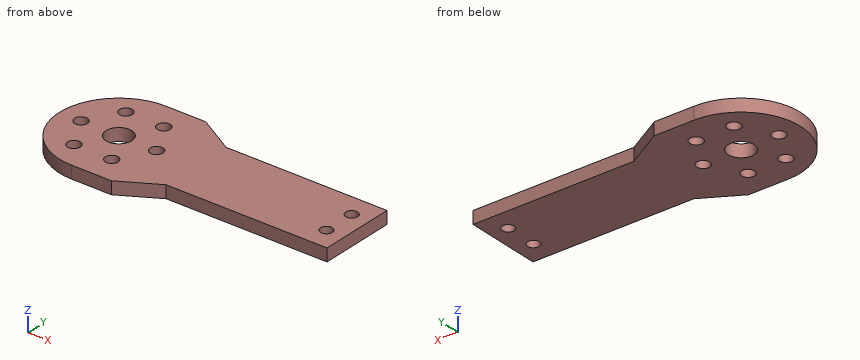
```python
from build123d import *

# Parameters (mm, degrees)
CROQUIS1_R                      = 1.5
CROQUIS1_R_2                    = 3.25
SALIENTE_EXTRUIR1_DEPTH         = 3.175
TALADRO_DE_MARGEN_PARA_41_D     = 3.2639
TALADRO_DE_MARGEN_PARA_41_DEPTH = 10
TALADRO_DE_MARGEN_PARA_41_TIP   = 0.980574487


with BuildPart() as part:
    # Croquis1 → Saliente-Extruir1 (new body)
    with BuildSketch(Plane.XY.offset(86.203907482)):
        with BuildLine():
            Line((0, -15), (10, -15))
            Line((10, -15), (19.474317917, -9.53))
            Line((19.474317917, -9.53), (60, -9.53))
            Line((60, -9.53), (60, 9.53))
            Line((60, 9.53), (19.474317917, 9.53))
            Line((19.474317917, 9.53), (10, 15))
            Line((10, 15), (0, 15))
            ThreePointArc((0, 15), (-15, 0), (0, -15))
        make_face()
        with Locations((55.5, 4)):
            Circle(CROQUIS1_R, mode=Mode.SUBTRACT)
        Circle(CROQUIS1_R_2, mode=Mode.SUBTRACT)
        with Locations((55.5, -4)):
            Circle(CROQUIS1_R, mode=Mode.SUBTRACT)
    extrude(amount=SALIENTE_EXTRUIR1_DEPTH)

    # Taladro de margen para #41
    with Locations(Plane.XY.offset(89.378907482)):
        with Locations((4.765, 8.253222098), (9.53, 0), (4.765, -8.253222098), (-4.765, -8.253222098), (-9.53, 0), (-4.765, 8.253222098)):
            Hole(TALADRO_DE_MARGEN_PARA_41_D / 2, depth=TALADRO_DE_MARGEN_PARA_41_DEPTH)
            with Locations((0, 0, -(TALADRO_DE_MARGEN_PARA_41_DEPTH + TALADRO_DE_MARGEN_PARA_41_TIP / 2))):  # 118° drill point
                Cone(0, TALADRO_DE_MARGEN_PARA_41_D / 2, TALADRO_DE_MARGEN_PARA_41_TIP, mode=Mode.SUBTRACT)


solid = part.part
```
For this review, take the finished solid that the model builds, in its own axes (mm). Coordinates: 2 decimals unless noted, no trailing zeros. Write each loop counter-clockwise with the first axis right and the second up, starting at its lowest first coordinate (ties: lowest second). Pieces come first, ordered by that corner, then holes. Notation, with made-up numbers: (58.25, 82.25) - (94.25, 82.25) arc R21 ccw to (94.25, 94.25) - close; hole circle Ø4 at (13.5, 84). An arc over 180 degrees is marked (long way). Put each result on its own line as item: value.
1. Add section D-D, the plane y = -4. Give the boundary of the cut face in (x, z), then the cut area to 3 significant figures.
Values found:
outline: (-14.46, 86.2) - (54, 86.2) - (54, 89.38) - (-14.46, 89.38) - close; (57, 86.2) - (60, 86.2) - (60, 89.38) - (57, 89.38) - close
area: 227 mm²
2. Add section C-C, the plane x = -9.53. Give the boundary of the cut face in (y, z).
Values found:
outline: (-11.58, 86.2) - (-1.63, 86.2) - (-1.63, 89.38) - (-11.58, 89.38) - close; (1.63, 86.2) - (11.58, 86.2) - (11.58, 89.38) - (1.63, 89.38) - close
3. Add section A-A, the plane y = 0. Give the boundary of the cut face in (x, z).
Values found:
outline: (-15, 86.2) - (-11.16, 86.2) - (-11.16, 89.38) - (-15, 89.38) - close; (-7.9, 86.2) - (-3.25, 86.2) - (-3.25, 89.38) - (-7.9, 89.38) - close; (3.25, 86.2) - (7.9, 86.2) - (7.9, 89.38) - (3.25, 89.38) - close; (11.16, 86.2) - (60, 86.2) - (60, 89.38) - (11.16, 89.38) - close
4. Wall thickness on probe 1 along Y at (x, z) = (55, 87.75); probe 2 along X at (y, z) = (-9.75, 87.3); probe 3 along X at (y, z) = (1, 88.7): over which ranges is each line inside the solid? List them lowest first.
Values found:
probe 1: -9.53 to -5.41, -2.59 to 2.59, 5.41 to 9.53
probe 2: -11.4 to -5.42, -4.11 to 4.11, 5.42 to 19.09
probe 3: -14.97 to -10.82, -8.24 to -3.09, 3.09 to 8.24, 10.82 to 60
5. For pin 1 (5 mm diameter, centred on x = 0, y = 0, fed in from -Z); pin 2 (1.5 mm diameter, centred on y = -11.5, z = 89, fed in from -X); pin 3 (1 mm diameter, centred on y = -11, z = 87, fed in from -X), all flat-tipped, find the tip position at first contact; note any pin that passes through.
Values found:
pin 1: through
pin 2: x = -10.46
pin 3: x = -10.71
6. Add section B-B, the plane x = 55.5. Give the boundary of the cut face in (y, z).
Values found:
outline: (-9.53, 86.2) - (-5.5, 86.2) - (-5.5, 89.38) - (-9.53, 89.38) - close; (-2.5, 86.2) - (2.5, 86.2) - (2.5, 89.38) - (-2.5, 89.38) - close; (5.5, 86.2) - (9.53, 86.2) - (9.53, 89.38) - (5.5, 89.38) - close
